```python
from build123d import *

# Parameters (mm, degrees)
SKETCH1_W           = 12.500000000000002
SKETCH1_H           = 25.399999999999995
BOSS_EXTRUDE1_DEPTH = 3.175
FILLET1_R           = 2.5
BOSS_EXTRUDE2_START = 1.95
BOSS_EXTRUDE2_DEPTH = 1.95
FILLET2_R           = 0.5


with BuildPart() as part:
    # Sketch1 → Boss-Extrude1 (new body)
    with BuildSketch(Plane.XY):
        with Locations((6.250000000000001, 12.699999999999998)):
            Rectangle(SKETCH1_W, SKETCH1_H)
        with BuildLine():
            Line((4.325, 4.875000000000003), (9.325, 4.874999999999999))
            ThreePointArc((9.325, 4.874999999999999), (11.025, 3.1750000000000007), (9.325, 1.474999999999999))
            Line((9.325, 1.474999999999999), (4.325, 1.4750000000000023))
            ThreePointArc((4.325, 1.4750000000000023), (2.625, 3.1750000000000025), (4.325, 4.875000000000003))
        make_face(mode=Mode.SUBTRACT)
        with BuildLine():
            Line((4.325, 23.925000000000004), (9.325, 23.925000000000004))
            ThreePointArc((9.325, 23.925000000000004), (11.025000000000002, 22.225), (9.325, 20.525))
            Line((9.325, 20.525), (4.325, 20.525))
            ThreePointArc((4.325, 20.525), (2.624999999999994, 22.224999999999998), (4.325, 23.925000000000004))
        make_face(mode=Mode.SUBTRACT)
    extrude(amount=BOSS_EXTRUDE1_DEPTH)

    # Fillet1
    fillet1_edges = [part.edges().sort_by_distance(p)[0] for p in [
        (0, 25.4, 1.5875),
        (12.5, 25.4, 1.5875),
        (12.5, 0, 1.5875),
        (0, 0, 1.5875),
    ]]
    fillet(fillet1_edges, radius=FILLET1_R)

    # Sketch2 → Boss-Extrude2 (add)
    with BuildSketch(Plane.XY.offset(3.175).offset(BOSS_EXTRUDE2_START)):
        with BuildLine():
            Line((0, 22.9), (0, 2.5))
            ThreePointArc((0, 2.5), (0.7322330470336307, 0.7322330470336313), (2.5, 0))
            Line((2.5, 0), (2.5, 1.5))
            ThreePointArc((2.5, 1.5), (1.7928932188134532, 1.7928932188134517), (1.5, 2.4999999999999987))
            Line((1.5, 2.4999999999999987), (1.5000000000000004, 22.9))
            ThreePointArc((1.5000000000000004, 22.9), (1.7928932188134499, 23.60710678118655), (2.5, 23.900000000000002))
            Line((2.5, 23.900000000000002), (2.5, 25.4))
            ThreePointArc((2.5, 25.4), (0.7322330470336313, 24.667766952966367), (0, 22.9))
        make_face()
    extrude(amount=-BOSS_EXTRUDE2_DEPTH)

    # Fillet2
    fillet2_edges = [part.edges().sort_by_distance(p)[0] for p in [
        (2.5, 25.4, 4.15),
        (2.5, 0, 4.15),
        (2.5, 1.5000000000000002, 4.15),
        (2.5, 23.900000000000002, 4.15),
    ]]
    fillet(fillet2_edges, radius=FILLET2_R)


solid = part.part
```
Check sheet for the modelled part. Datum: model origin and axes. Units: mm. A direction names the side the tool comes from. Give positions to 0.01 mm unless a question says otherwise; leave off trailing zeros. Loops run counter-clockwise (first coordinate to the right, second up) from the corner with the lowest first, then second, coordinate; pieces in that order, holes last. Notation, with made-up numbers: M 21.25,5 L 74.25,5 A8 cw 74.25,14 Z; hole C -34.5,12 d11. An arc over 180 degrees is marked long. Answer in a Markdown table with one row per item.
1) Cross-section at C-C (z = 0.55). Enter the section's corners in (x, y) (3 decimals), plus the area to 3 significant figures.
Solutions:
| item | result |
|---|---|
| outline | M 0,2.5 A2.5 ccw 2.5,0 L 10,0 A2.5 ccw 12.5,2.5 L 12.5,22.9 A2.5 ccw 10,25.4 L 2.5,25.4 A2.5 ccw 0,22.9 Z; hole M 4.325,1.475 L 9.325,1.475 A1.7 ccw 9.325,4.875 L 4.325,4.875 A1.7 ccw Z; hole M 4.325,20.525 L 9.325,20.525 A1.7 ccw 9.325,23.925 L 4.325,23.925 A1.7 ccw Z |
| area | 260 mm^2 |
2) Cross-section at D-D (z = 4.75). Enter the section's corners in (x, y) (1 decimal), plus the area to 3 significant figures.
Solutions:
| item | result |
|---|---|
| outline | M 0,2.5 A2.5 ccw 1.9,0.1 A0.5 ccw 2.5,0.6 L 2.5,1.1 A0.5 ccw 2.2,1.6 A1 cw 1.5,2.5 L 1.5,22.9 A1 cw 2.2,23.8 A0.5 ccw 2.5,24.3 L 2.5,24.8 A0.5 ccw 1.9,25.3 A2.5 ccw 0,22.9 Z |
| area | 38.6 mm^2 |
3) Cross-section at B-B (x = 8.5). Enter the section's corners in (y, z) (3 decimals), plus the area to 3 significant figures.
Solutions:
| item | result |
|---|---|
| outline | M 0,0 L 1.475,0 L 1.475,3.175 L 0,3.175 Z; M 4.875,0 L 20.525,0 L 20.525,3.175 L 4.875,3.175 Z; M 23.925,0 L 25.4,0 L 25.4,3.175 L 23.925,3.175 Z |
| area | 59.1 mm^2 |
4) Cross-section at A-A (y = 22). Enter the section's corners in (x, z) (3 decimals), plus the area to 3 significant figures.
Solutions:
| item | result |
|---|---|
| outline | M 0,0 L 2.64,0 L 2.64,3.175 L 1.5,3.175 L 1.5,5.125 L 0,5.125 Z; M 11.01,0 L 12.5,0 L 12.5,3.175 L 11.01,3.175 Z |
| area | 16.0 mm^2 |
5) Thickness scan on line 1 (Y direction, x = 4.5, z = 1.55) (3 decimals); line 2 (Y direction, x = 10.25, z = 1.15); line 3 (Z direction, x = 7, y = 8) (3 decimals). Record the ranges inside material, lowest first.
Solutions:
| item | result |
|---|---|
| line 1 | y = 0 to 1.475, 4.875 to 20.525, 23.925 to 25.4 |
| line 2 | y = 0.01 to 1.75, 4.6 to 20.8, 23.65 to 25.39 |
| line 3 | z = 0 to 3.175 |
6) Depth check by flat-ended pin: pin 1 (2 mm diameter, centred on x = 6, y = 16, fed in from +Z) (3 decimals); pin 2 (2 mm diameter, centred on x = 2, z = 1, fed in from -Y). Enter the tip coordinate at first touch or a pass-through.
Solutions:
| item | result |
|---|---|
| pin 1 | stops at z = 3.175 |
| pin 2 | stops at y = 0 |
7) Mould release check, pull along X, two halves, no side actions. Record for faces 1 (the face through (2.625, 22.188, 1.565)), 2 (the face through (1.5, 13, 4)), 3 (the face through (1, 13, 5.125)): released by +X, released by -X, zero draft, split by the parting line, or undercut.
Solutions:
| item | result |
|---|---|
| face 1 | undercut |
| face 2 | released by +X |
| face 3 | zero draft |
8) Tool access check on faces 4 (the face through (6, 13, 0)), 5 (the face through (1.7, 23.5, 4.2)), 6 (the face through (7, 1.475, 2)). Record the directions out of +Z, -Z, +X, -X, +Y, -Y that give a thin tool (end or side, any length) a straight path to the whole face; none if there is none.
Solutions:
| item | result |
|---|---|
| face 4 | -Z, +X, -X, +Y, -Y |
| face 5 | +Z, +X |
| face 6 | +Z, -Z |
